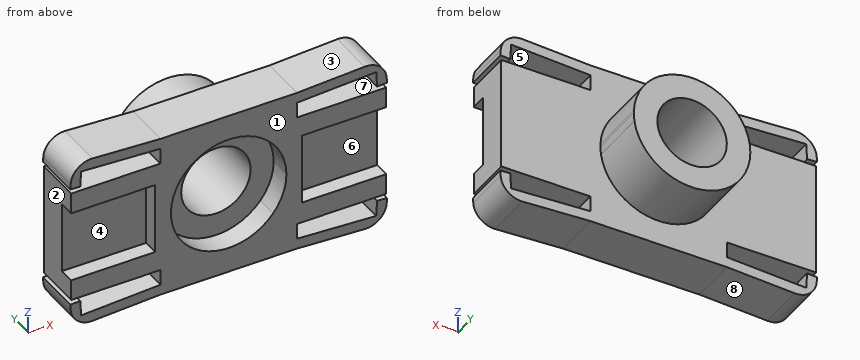
```python
from build123d import *
from build123d.topology import SkipClean

# Parameters (mm, degrees)
BOSS_EXTRU_1_DEPTH       = 4.5
BOSS_EXTRU_2_DEPTH       = 5.5
ENL_V_MAT_EXTRU_3_DEPTH  = 2.1
ENL_V_START              = -13.1
ESQUISSE7_R              = 3
ENL_V_MAT_EXTRU_4_DEPTH  = 13.1
ESQUISSE18_W             = 8
ESQUISSE18_H             = 6.792682927
ENL_V_MAT_EXTRU_5_DEPTH  = 1.5
ESQUISSE19_W             = 8
ESQUISSE19_H             = 6.792682927
ENL_V_MAT_EXTRU_6_DEPTH  = 1.5
BOSS_EXTRU_11_DEPTH      = 4.5
ESQUISSE25_W             = 0.947664044
ESQUISSE25_H             = 4.5
BOSS_EXTRU_12_DEPTH      = 1.5
CONG_16_R                = 2
BOSS_EXTRU_16_DEPTH      = 1
ENL_V_MAT_EXTRU_7_DEPTH  = 0.25
CONG_16_OF_SYM_TRIE4_R   = 2
SYM_TRIE5_DEPTH          = 4.5
ESQUISSE34_W             = 0.75
ESQUISSE34_H             = 11.333514389
ENL_V_MAT_EXTRU_10_DEPTH = 36
ESQUISSE35_R             = 5.54436651
ESQUISSE35_R_2           = 3
BOSS_EXTRU_19_DEPTH      = 5.5
ESQUISSE36_W             = 0.010434814
ESQUISSE36_H             = 5.5
ENL_V_MAT_EXTRU_11_DEPTH = 0.25
BOSS_EXTRU_20_DEPTH      = 5.5
ESQUISSE38_W             = 0.005685697
ESQUISSE38_H             = 5.5
ENL_V_MAT_EXTRU_12_DEPTH = 36
ESQUISSE39_R             = 3.307933445
ENL_V_MAT_EXTRU_13_DEPTH = 5.5
ENL_V_START_2            = -36
ESQUISSE40_R             = 3.307933445
ENL_V_MAT_EXTRU_14_DEPTH = 36


with BuildPart() as part:
    # Esquisse1 → Boss.-Extru.1 (new body)
    with BuildSketch(Plane(origin=(0, 0, 0), x_dir=(1, 0, 0), z_dir=(0, 1, 0))):
        Polygon((21.5, 0), (21.5, 2.5), (8.5, 2.5), (8.5, 0), (0, 0), (0, -10.792682927), (8.5, -10.792682927), (8.5, -13.292682927), (21.5, -13.292682927), (21.5, -10.792682927), (30, -10.792682927), (30, 0), align=None)
    extrude(amount=BOSS_EXTRU_1_DEPTH)

    # Esquisse2 → Boss.-Extru.2 (add)
    with BuildSketch(Plane(origin=(0, 4.5, 0), x_dir=(1, 0, 0), z_dir=(0, 1, 0))):
        with BuildLine():
            ThreePointArc((20.55, -5.396341463), (16.884536839, -0.176090425), (10.729812288, -1.851204385))
            Line((10.729812288, -1.851204385), (12.691790426, -3.480051151))
            ThreePointArc((12.691790426, -3.480051151), (16.018668562, -2.574584145), (18, -5.396341463))
            ThreePointArc((18, -5.396341463), (17.821757318, -6.415010025), (17.308209574, -7.312631776))
            Line((17.308209574, -7.312631776), (19.270187712, -8.941478542))
            ThreePointArc((19.270187712, -8.941478542), (20.220251038, -7.280878303), (20.55, -5.396341463))
        make_face()
        with BuildLine():
            Line((12.691790426, -3.480051151), (10.729812288, -1.851204385))
            ThreePointArc((10.729812288, -1.851204385), (11.454862922, -9.666529176), (19.270187712, -8.941478542))
            Line((19.270187712, -8.941478542), (17.308209574, -7.312631776))
            ThreePointArc((17.308209574, -7.312631776), (13.083709687, -7.704551038), (12.691790426, -3.480051151))
        make_face()
        with BuildLine():
            ThreePointArc((20.55, -5.396341463), (16.884536839, -0.176090425), (10.729812288, -1.851204385))
            Line((10.729812288, -1.851204385), (12.691790426, -3.480051151))
            ThreePointArc((12.691790426, -3.480051151), (16.018668562, -2.574584145), (18, -5.396341463))
            ThreePointArc((18, -5.396341463), (17.821757318, -6.415010025), (17.308209574, -7.312631776))
            Line((17.308209574, -7.312631776), (19.270187712, -8.941478542))
            ThreePointArc((19.270187712, -8.941478542), (20.220251038, -7.280878303), (20.55, -5.396341463))
        make_face()
        with BuildLine():
            Line((12.691790426, -3.480051151), (10.729812288, -1.851204385))
            ThreePointArc((10.729812288, -1.851204385), (11.454862922, -9.666529176), (19.270187712, -8.941478542))
            Line((19.270187712, -8.941478542), (17.308209574, -7.312631776))
            ThreePointArc((17.308209574, -7.312631776), (13.083709687, -7.704551038), (12.691790426, -3.480051151))
        make_face()
    extrude(amount=BOSS_EXTRU_2_DEPTH)

    # Esquisse5 → Enlèv. mat.-Extru.3 (cut)
    with BuildSketch(Plane.XZ):
        with BuildLine():
            ThreePointArc((20.5, 5.396341463), (16.86755903, 10.569563213), (10.768282447, 8.90954037))
            Line((10.768282447, 8.90954037), (19.231717553, 1.883142557))
            ThreePointArc((19.231717553, 1.883142557), (20.17322175, 3.528782433), (20.5, 5.396341463))
        make_face()
        with BuildLine():
            Line((19.231717553, 1.883142557), (10.768282447, 8.90954037))
            ThreePointArc((10.768282447, 8.90954037), (11.486801094, 1.164623911), (19.231717553, 1.883142557))
        make_face()
        with BuildLine():
            ThreePointArc((20.5, 5.396341463), (16.86755903, 10.569563213), (10.768282447, 8.90954037))
            Line((10.768282447, 8.90954037), (19.231717553, 1.883142557))
            ThreePointArc((19.231717553, 1.883142557), (20.17322175, 3.528782433), (20.5, 5.396341463))
        make_face()
        with BuildLine():
            Line((19.231717553, 1.883142557), (10.768282447, 8.90954037))
            ThreePointArc((10.768282447, 8.90954037), (11.486801094, 1.164623911), (19.231717553, 1.883142557))
        make_face()
    extrude(amount=-ENL_V_MAT_EXTRU_3_DEPTH, mode=Mode.SUBTRACT)

    # Esquisse7 → Enlèv. mat.-Extru.4 (cut)
    with BuildSketch(Plane(origin=(0, 4.5, 0), x_dir=(1, 0, 0), z_dir=(0, 1, 0)).offset(ENL_V_START)):
        with Locations(Location((15, -5.396341463, 0), (0, 0, 90))):
            Circle(ESQUISSE7_R)
    extrude(amount=ENL_V_MAT_EXTRU_4_DEPTH, mode=Mode.SUBTRACT)

    # Esquisse18 → Enlèv. mat.-Extru.5 (cut)
    with BuildSketch(Plane.XZ):
        with Locations((26, 5.396341464)):
            Rectangle(ESQUISSE18_W, ESQUISSE18_H)
    extrude(amount=-ENL_V_MAT_EXTRU_5_DEPTH, mode=Mode.SUBTRACT)

    # Esquisse19 → Enlèv. mat.-Extru.6 (cut)
    with BuildSketch(Plane.XZ):
        with Locations((4, 5.396341464)):
            Rectangle(ESQUISSE19_W, ESQUISSE19_H)
    extrude(amount=-ENL_V_MAT_EXTRU_6_DEPTH, mode=Mode.SUBTRACT)

    # Esquisse23 → Boss.-Extru.11 (add)
    with BuildSketch(Plane(origin=(0, 4.5, 0), x_dir=(1, 0, 0), z_dir=(0, 1, 0))):
        Polygon((21.5, 2.5), (30, 2.945466124), (30, 1.945466124), (21.5, 1.5), align=None)
    boss_extru_11 = extrude(amount=-BOSS_EXTRU_11_DEPTH)

    # Esquisse25 → Boss.-Extru.12 (add)
    with BuildSketch(Plane(origin=(-0.019506723, 0, -0.372210441), x_dir=(0.998629534754574, 0, -0.05233595624294039), z_dir=(0.05233595624294039, 0, 0.9986295347545742))):
        with Locations((29.586871851, 2.25)):
            Rectangle(ESQUISSE25_W, ESQUISSE25_H)
    boss_extru_12 = extrude(amount=BOSS_EXTRU_12_DEPTH)

    # Congé16
    cong_16_edges = [part.edges().sort_by_distance(p)[0] for p in [
        (30, 2.25, -2.945466124),
    ]]
    fillet(cong_16_edges, radius=CONG_16_R)

    # Esquisse3D3 → Boss.-Extru.16 (add)
    with SkipClean():  # the faces are left unmerged after this step: merging them gives an invalid solid
        with BuildSketch(Plane(origin=(15, 4.5, 5.646341463), x_dir=(0.9055110385022749, 0.42432270638104186, 1.6236855905047217e-15), z_dir=(0, 0, -1))):
            Polygon((0, 0), (21.900590549, 10.262622385), (26.709658048, 0), (4.809067498, -10.262622385), align=None)
        extrude(amount=BOSS_EXTRU_16_DEPTH)

    # Esquisse29 → Enlèv. mat.-Extru.7 (cut)
    with BuildSketch(Plane.XY.offset(5.646341463)):
        Polygon((17.989565186, 4.5), (17.989565186, 10), (20.54436651, 10), (20.54436651, 4.5), (30, 4.5), (39.185890197, 4.5), (39.185890197, 15.833514389), (15, 15.833514389), (15, 4.5), align=None)
    extrude(amount=-ENL_V_MAT_EXTRU_7_DEPTH, mode=Mode.SUBTRACT)

    # Symétrie4: Boss.-Extru.11, Boss.-Extru.12 across plane
    add(boss_extru_11.mirror(Plane.XY.offset(5.396341463)))
    add(boss_extru_12.mirror(Plane.XY.offset(5.396341463)))

    # Congé16 of Symétrie4
    cong_16_of_sym_trie4_edges = [part.edges().sort_by_distance(p)[0] for p in [
        (30, 2.25, 13.738149051),
    ]]
    fillet(cong_16_of_sym_trie4_edges, radius=CONG_16_OF_SYM_TRIE4_R)

    # Symétrie5: read off the stored shape, not the designer's step
    # Symétrie5 outline → Symétrie5 (add)
    with BuildSketch(Plane(origin=(0, 0, 0), x_dir=(1, 0, 0), z_dir=(0, 1, 0))):
        with BuildLine():
            Line((8.5, -13.292682927), (8.5, -12.292682927))
            Line((8.5, -12.292682927), (0.946365303, -12.688552147))
            Line((0.946365303, -12.688552147), (0.867861369, -11.190607845))
            Line((0.867861369, -11.190607845), (-0.078503934, -11.240204749))
            Line((-0.078503934, -11.240204749), (-0.052407681, -11.738150929))
            ThreePointArc((-0.052407681, -11.738150929), (0.606590176, -13.119768667), (2.049523301, -13.630738086))
            Line((2.049523301, -13.630738086), (8.5, -13.292682927))
        make_face()
        with BuildLine():
            Line((0.946365303, 1.89586922), (8.5, 1.5))
            Line((8.5, 1.5), (8.5, 2.5))
            Line((8.5, 2.5), (2.049523301, 2.838055159))
            ThreePointArc((2.049523301, 2.838055159), (0.606590176, 2.327085741), (-0.052407681, 0.945468002))
            Line((-0.052407681, 0.945468002), (-0.078503934, 0.447521822))
            Line((-0.078503934, 0.447521822), (0.867861369, 0.397924918))
            Line((0.867861369, 0.397924918), (0.946365303, 1.89586922))
        make_face()
    extrude(amount=SYM_TRIE5_DEPTH)

    # Esquisse34 → Enlèv. mat.-Extru.10 (cut)
    with SkipClean():  # the faces are left unmerged after this step: merging them gives an invalid solid
        with BuildSketch(Plane.ZY.offset(-15)):
            with Locations((5.021341463, 10.166757195)):
                Rectangle(ESQUISSE34_W, ESQUISSE34_H)
        extrude(amount=-ENL_V_MAT_EXTRU_10_DEPTH, mode=Mode.SUBTRACT)

    # Esquisse35 → Boss.-Extru.19 (add)
    with BuildSketch(Plane(origin=(0, 4.5, 0), x_dir=(1, 0, 0), z_dir=(0, 1, 0))):
        with Locations((15, -5.396341463)):
            Circle(ESQUISSE35_R)
        with Locations(Location((15, -5.396341463, 0), (0, 0, 90))):
            Circle(ESQUISSE35_R_2, mode=Mode.SUBTRACT)
    extrude(amount=BOSS_EXTRU_19_DEPTH)

    # Esquisse36 → Enlèv. mat.-Extru.11 (cut)
    with SkipClean():  # the faces are left unmerged after this step: merging them gives an invalid solid
        with BuildSketch(Plane(origin=(0, 0, 5.396341463), x_dir=(-1, 0, 0), z_dir=(0, 0, -1))):
            with Locations((-17.994782593, 7.25)):
                Rectangle(ESQUISSE36_W, ESQUISSE36_H)
        extrude(amount=-ENL_V_MAT_EXTRU_11_DEPTH, mode=Mode.SUBTRACT)

    # Esquisse37 → Boss.-Extru.20 (add)
    with SkipClean():  # the faces are left unmerged after this step: merging them gives an invalid solid
        with BuildSketch(Plane(origin=(0, 4.5, 0), x_dir=(1, 0, 0), z_dir=(0, 1, 0))):
            with BuildLine():
                Line((17.989565186, -5.646341463), (18, -5.646341463))
                Line((18, -5.646341463), (18, -5.396341463))
                ThreePointArc((18, -5.396341463), (17.997390161, -5.521450301), (17.989565186, -5.646341463))
            make_face()
        extrude(amount=BOSS_EXTRU_20_DEPTH)

    # Esquisse38 → Enlèv. mat.-Extru.12 (cut)
    with SkipClean():  # the faces are left unmerged after this step: merging them gives an invalid solid
        with BuildSketch(Plane.XY.offset(4.646341463)):
            with Locations((20.496247985, 7.25)):
                Rectangle(ESQUISSE38_W, ESQUISSE38_H)
        extrude(amount=-ENL_V_MAT_EXTRU_12_DEPTH, mode=Mode.SUBTRACT)

    # Esquisse39 → Enlèv. mat.-Extru.13 (cut)
    with BuildSketch(Plane(origin=(0, 4.5, 0), x_dir=(1, 0, 0), z_dir=(0, 1, 0))):
        with Locations(Location((15, -5.396341463, 0), (0, 0, 270))):
            Circle(ESQUISSE39_R)
    extrude(amount=ENL_V_MAT_EXTRU_13_DEPTH, mode=Mode.SUBTRACT)

    # Esquisse40 → Enlèv. mat.-Extru.14 (cut)
    with BuildSketch(Plane(origin=(0, 4.5, 0), x_dir=(1, 0, 0), z_dir=(0, 1, 0)).offset(ENL_V_START_2)):
        with Locations(Location((15, -5.396341463, 0), (0, 0, 90))):
            Circle(ESQUISSE40_R)
    extrude(amount=ENL_V_MAT_EXTRU_14_DEPTH, mode=Mode.SUBTRACT)


solid = part.part
```
Verification items for the finished model (mm, model axes). Face numbers are marked on the shaded views. A direction names the side the tool comes from. Give positions to 0.01 mm unless a question says otherwise; leave off trailing zeros. Loops run counter-clockwise (first coordinate to the right, second up) from the corner with the lowest first, then second, coordinate; pieces in that order, holes last.
1. Go/stop test with flat-tipped pins: pin 1 Ø1 at (y, z) = (8, 2) entering from -X; pin 2 Ø5.5 at (x, z) = (27.5, 5) entering from -Y; pin 3 Ø2 at (y, z) = (3, 8) entering from +X; pin 4 Ø1.5 at (x, z) = (11.5, 0.5) entering from -Y. Record where each tip stops, or that it passes through.
2. Section check B-B, the plane y = 7.75. Enter the section's corners in (x, z), then the cut area to 3 significant figures.
3. Section check A-A, the plane x = 15. Enter the section's corners in (y, z).
4. Mould release check, pull along X, two halves, no side actions. Record for the marked faces 1, 2 and 3: released by +X, released by -X, zero draft, split by the parting line, or undercut.
5. Section check C-C, the plane x = 3. Enter the section's corners in (y, z), then the cut area to 3 significant figures.
6. Set-up check for the marked faces 4, 5, 6, 7 and 8: record each of +Z, -Z, +X, -X, +Y, -Y from which the full face is reachable in a straight line by a thin tool's end or side.
7. Thickness scan on line 1 (Z direction, x = 15, y = 6.25); line 2 (Z direction, x = 15, y = 3.5); line 3 (Y direction, x = 3.5, z = 3.75). Record the ranges inside material, lowest first.
Geometry says:
1. pin 1: stops at x = 10.27
1. pin 2: stops at y = 1.5
1. pin 3: stops at x = 30
1. pin 4: stops at y = 0
2. outline: (20.49, 4.61) - (20.49, 4.65) arc R5.54 ccw to (20.54, 5.4) - (20.54, 5.65) arc R5.55 ccw (long way) to start; hole circle Ø6.62 at (15, 5.4)
2. area: 62.4 mm2
3. outline: (0, -2.5) - (4.5, -2.5) - (4.5, -0.15) - (10, -0.15) - (10, 2.09) - (2.1, 2.09) - (2.1, -0.1) - (0, -0.1) - close; (0, 10.9) - (2.1, 10.9) - (2.1, 8.7) - (10, 8.7) - (10, 10.95) - (4.5, 10.95) - (4.5, 13.29) - (0, 13.29) - close
4. face 1: zero draft
4. face 2: released by -X
4. face 3: undercut
5. outline: (0, -2.79) - (4.5, -2.79) - (4.5, -1.79) - (0, -1.79) - close; (0, 0) - (4.5, 0) - (4.5, 10.79) - (0, 10.79) - (0, 8.79) - (1.5, 8.79) - (1.5, 2) - (0, 2) - close; (0, 12.58) - (4.5, 12.58) - (4.5, 13.58) - (0, 13.58) - close
5. area: 47.4 mm2
6. face 4: -X, -Y
6. face 5: +Y, -Y
6. face 6: +X, -Y
6. face 7: +X, +Y, -Y
6. face 8: -Z, +Y, -Y
7. line 1: z = -0.15 to 2.09, 8.7 to 10.95
7. line 2: z = -2.5 to 2.09, 8.7 to 13.29
7. line 3: y = 1.5 to 4.5
